Autodesk Inventor part; units mm, degrees
ref_plane "Work Plane1" through (0, 0, 0) normal (1, 0, 0) x (0, 1, 0)
ref_plane "XZ Plane" through (0, 0, 0) normal (0, 1, 0) x (-1, 0, 0)
ref_plane "XY Plane" through (0, 0, 0) normal (0, 0, 1) x (1, 0, 0)
sketch "Sketch1" plane through (0, 0, 0) normal (1, 0, 0) x (0, 1, 0)
  circle A0 centre (0, 0) radius 11
  dimension "d0" = 22
extrude "Extrusion1" add sketch "Sketch1" along normal mid plane 46
sketch "Sketch3" plane through (23, 0, 0) normal (1, 0, 0) x (0, 0, -1)
  circle A0 centre (0, 0) radius 7.5
  dimension "d3" = 15
extrude "Extrusion2" add sketch "Sketch3" along normal blind 18
thread "Thread1"
ref_plane "Work Plane1" through (0, 0, 0) normal (1, 0, 0) x (0, 1, 0)
mirror "Mirror2" about plane through (0, 0, 0) normal (1, 0, 0) of "Extrusion2"
properties part number "5. PlateSpacers" material "Silicon Nitride"
Design review of the part built by this model. Coordinates are the model's own, in mm. A direction names the side the tool comes from. Coordinates: 2 decimals unless noted, no trailing zeros. Order: outer loops, then holes, each group sorted by start corner. A loop starts at its lowest first (then second) coordinate and runs counter-clockwise, first axis right, second up. Notation, with made-up numbers: (57.25, 52.5) - (78.25, 52.5) arc R23 ccw to (78.25, 74.5) - close; hole circle Ø6 at (-23, 6.5). An arc over 180 degrees is marked (long way). One line per question, with ' | ' between items.
Q1. Consider section C-C, the plane x = 6. Give the boundary of the cut face in (y, z).
Answer key:
outline: circle Ø22 at (0, 0)
Q2. To check wall thickness, follow line 1 along X through (y, z) = (-6.25, -9); line 2 along Z through (x, y) = (-18.5, 2.5); line 3 along Z through (x, y) = (4.5, 7). State the ranges of each line that lie inside material, in increasing order.
Answer key:
line 1: x = -23 to 23 | line 2: z = -10.71 to 10.71 | line 3: z = -8.49 to 8.49
Q3. Clearance check with flat-ended pins moving along their axes: pin 1 Ø3 at (y, z) = (3.5, -8.5) entering from +X; pin 2 Ø10 at (x, z) = (5.5, -7) entering from +Y; pin 3 Ø1 at (x, y) = (5.5, 4) entering from +Z. State where each tip first meets the part, or that it passes through.
Answer key:
pin 1: stops at x = 23 | pin 2: stops at y = 10.82 | pin 3: stops at z = 10.43
Q4. For faces 1 (the cylindrical face through (31.874, -0.33, 7.493)), 2 (the cylindrical face through (-31.874, 0.33, 7.493)), 3 (the flat face through (41, 0, 0)), list the 3-axis set-ups (+Z, -Z, +X, -X, +Y, -Y) from which the entire face can be reached by the end or side of a thin tool; tool diameter is ignored.
Answer key:
face 1: +X | face 2: -X | face 3: +Z, -Z, +X, +Y, -Y
Q5. Consider section D-D, the plane x = -31. Give the boundary of the cut face in (y, z).
Answer key:
outline: circle Ø15 at (0, 0)
Q6. Consider section A-A, the plane y = 0. Give the boundary of the cut face in (x, z), then the cut area to 3 significant figures.
Answer key:
outline: (-41, -7.5) - (-23, -7.5) - (-23, -11) - (23, -11) - (23, -7.5) - (41, -7.5) - (41, 7.5) - (23, 7.5) - (23, 11) - (-23, 11) - (-23, 7.5) - (-41, 7.5) - close | area: 1,550 mm2
